```python
from build123d import *

# Parameters (mm, degrees)
F0_R     = 2
F0_R_2   = 2.5
F1_DEPTH = 2
F2_R     = 2
F3_R     = 5
F4_R     = 12
F5_R     = 5
F6_R     = 16


with BuildPart() as f1:
    # F0 (on Top) → F1 (new body)
    with BuildSketch(Plane.XY):
        Polygon((-40.6955056692, 2.5), (-31.6955056692, 2.5), (-31.6955056692, 9.2036510807), (-65, 42.5081454115), (-65, 34.5), (-65, 2.5), align=None)
        with Locations((-40.6955056692, 11.5)):
            Circle(F0_R, mode=Mode.SUBTRACT)
        with Locations((-59, 25.5)):
            Circle(F0_R, mode=Mode.SUBTRACT)
        with BuildLine():
            Line((-44, -28.5), (-26, -28.5))
            Line((-26, -28.5), (-26, -0.5))
            Line((-26, -0.5), (-28.6955056692, -0.5))
            ThreePointArc((-28.6955056692, -0.5), (-30.8168260127, 0.3786796564), (-31.6955056692, 2.5))
            Line((-31.6955056692, 2.5), (-40.6955056692, 2.5))
            Line((-40.6955056692, 2.5), (-65, 2.5))
            ThreePointArc((-65, 2.5), (-65.8786796564, 0.3786796564), (-68, -0.5))
            Line((-68, -0.5), (-68, -3))
            Line((-68, -3), (-66, -3))
            Line((-66, -3), (-66, -10))
            Line((-66, -10), (-68, -10))
            Line((-68, -10), (-68, -19.5))
            Line((-68, -19.5), (-55, -19.5))
            Line((-55, -19.5), (-44, -28.5))
        make_face()
        Polygon((-74, -3), (-68, -3), (-68, -0.5), (-72, -0.5), (-74, -0.5), align=None)
        with BuildLine():
            Line((-81, -19.5), (-68, -19.5))
            Line((-68, -19.5), (-68, -10))
            Line((-68, -10), (-71.5, -10))
            Line((-71.5, -10), (-71.5, -13.5))
            ThreePointArc((-71.5, -13.5), (-74, -16), (-76.5, -13.5))
            Line((-76.5, -13.5), (-76.5, -8.9494897428))
            ThreePointArc((-76.5, -8.9494897428), (-77.2267021942, -5.1441264992), (-74, -3))
            Line((-74, -3), (-74, -0.5))
            Line((-74, -0.5), (-81, -0.5))
            Line((-81, -0.5), (-81, -19.5))
        make_face()
        Polygon((-81, 2.5), (-81, -0.5), (-74, -0.5), (-72, -0.5), (-72, 10.5), (-86, 10.5), (-86, 2.5), align=None)
        with Locations((-79, 6.5)):
            Circle(F0_R, mode=Mode.SUBTRACT)
        with BuildLine():
            ThreePointArc((26, 24.5), (24.8284271247, 27.3284271247), (22, 28.5))
            Line((22, 28.5), (18.5, 28.5))
            Line((18.5, 28.5), (15, 28.5))
            ThreePointArc((15, 28.5), (12.1715728753, 27.3284271247), (11, 24.5))
            Line((11, 24.5), (11, 2.5))
            Line((11, 2.5), (11, 1.4913195046))
            ThreePointArc((11, 1.4913195046), (10, 0.4913195046), (9, 1.4913195046))
            Line((9, 1.4913195046), (9, 2.4990135962))
            Line((9, 2.4990135962), (9, 8.4837929157))
            Line((9, 8.4837929157), (-7.795591982, 28.5))
            Line((-7.795591982, 28.5), (-15.9371936145, 28.5))
            ThreePointArc((-15.9371936145, 28.5), (-16, 28.4990135962), (-16.0628063855, 28.5))
            Line((-16.0628063855, 28.5), (-21, 28.5))
            Line((-21, 28.5), (-21, 10.4990135962))
            Line((-21, 10.4990135962), (-21, 2.4990135962))
            ThreePointArc((-21, 2.4990135962), (-21.8516547202, 0.4050669496), (-23.9230750393, -0.5))
            ThreePointArc((-23.9230750393, -0.5), (-24, -0.5009864038), (-24.0769249607, -0.5))
            Line((-24.0769249607, -0.5), (-26, -0.5))
            Line((-26, -0.5), (-26, -28.5))
            Line((-26, -28.5), (-7, -28.5))
            Line((-7, -28.5), (9, -28.5))
            Line((9, -28.5), (10, -28.5))
            Line((10, -28.5), (11, -28.5))
            Line((11, -28.5), (22, -28.5))
            ThreePointArc((22, -28.5), (24.8284271247, -27.3284271247), (26, -24.5))
            Line((26, -24.5), (26, 24.5))
        make_face()
        with BuildLine():
            ThreePointArc((12.5, -18.5), (11.767766953, -20.267766953), (10, -21))
            ThreePointArc((10, -21), (8.232233047, -16.732233047), (12.5, -18.5))
        make_face(mode=Mode.SUBTRACT)
        with Locations((-7, -9.5)):
            Circle(F0_R_2, mode=Mode.SUBTRACT)
        with BuildLine():
            ThreePointArc((-14, 10.4990135962), (-16, 8.4990135962), (-18, 10.4990135962))
            ThreePointArc((-18, 10.4990135962), (-16, 12.4990135962), (-14, 10.4990135962))
        make_face(mode=Mode.SUBTRACT)
        with BuildLine():
            ThreePointArc((3, 10.4990135962), (1, 8.4990135962), (-1, 10.4990135962))
            ThreePointArc((-1, 10.4990135962), (1, 12.4990135962), (3, 10.4990135962))
        make_face(mode=Mode.SUBTRACT)
        with BuildLine():
            ThreePointArc((21, 14.5), (16.732233047, 12.732233047), (18.5, 17))
            ThreePointArc((18.5, 17), (20.267766953, 16.267766953), (21, 14.5))
        make_face(mode=Mode.SUBTRACT)
        with BuildLine():
            Line((-15.9371936145, 28.5), (-7.795591982, 28.5))
            Line((-7.795591982, 28.5), (-12.1697777844, 33.7129516447))
            ThreePointArc((-12.1697777844, 33.7129516447), (-17.7101007166, 35.1974767002), (-21, 30.4990135962))
            Line((-21, 30.4990135962), (-21, 28.5))
            Line((-21, 28.5), (-16.0628063855, 28.5))
            ThreePointArc((-16.0628063855, 28.5), (-17.3918310294, 31.9352609236), (-14, 30.4990135962))
            ThreePointArc((-14, 30.4990135962), (-14.5637526726, 29.1071825668), (-15.9371936145, 28.5))
        make_face()
    extrude(amount=F1_DEPTH)

    # F2
    f2_edges = [f1.edges().sort_by_distance(p)[0] for p in [
        (-72, 10.5, 1),
        (-86, 10.5, 1),
        (-86, 2.5, 1),
        (-81, 2.5, 1),
        (-72, -0.5, 1),
    ]]
    fillet(f2_edges, radius=F2_R)

    # F3
    f3_edges = [f1.edges().sort_by_distance(p)[0] for p in [
        (-65, 42.508145, 1),
    ]]
    fillet(f3_edges, radius=F3_R)

    # F4
    f4_edges = [f1.edges().sort_by_distance(p)[0] for p in [
        (-31.695506, 9.203651, 1),
        (9, 8.483793, 1),
    ]]
    fillet(f4_edges, radius=F4_R)

    # F5
    f5_edges = [f1.edges().sort_by_distance(p)[0] for p in [
        (-81, -19.5, 1),
    ]]
    fillet(f5_edges, radius=F5_R)

    # F6
    f6_edges = [f1.edges().sort_by_distance(p)[0] for p in [
        (-55, -19.5, 1),
        (-44, -28.5, 1),
    ]]
    fillet(f6_edges, radius=F6_R)


solid = f1.part
```
Input: part model. Units: mm. Frame: model coordinates. A direction names the side the tool comes from. Coordinates: 2 decimals unless noted, no trailing zeros. Write each loop counter-clockwise with the first axis right and the second up, starting at its lowest first coordinate (ties: lowest second). Pieces come first, ordered by that corner, then holes. Notation, with made-up numbers: M 33.25,58 L 58.25,58 A11 cw 58.25,74 Z; hole C 7,80.25 d8. An arc over 180 degrees is marked long. Use one line per item in the form item = value.
Q1. Section C-C (x = -79). Return loops of the section in (y, z), plus the area to 3 significant figures.
Answer below:
outline = M -18.5,0 L 4.5,0 L 4.5,2 L -18.5,2 Z; M 8.5,0 L 10.5,0 L 10.5,2 L 8.5,2 Z
area = 50.0 mm²
Q2. Section A-A (x = -59). Return loops of the section in (y, z).
Answer below:
outline = M -19.59,0 L 23.5,0 L 23.5,2 L -19.59,2 Z; M 27.5,0 L 35.34,0 L 35.34,2 L 27.5,2 Z
Q3. Section D-D (z = 1.3). Count the separate pieces of the cut face and the enclosed holes in it, plus the area to 3 significant figures.
Answer below:
separate_pieces = 1
enclosed_holes = 10
area = 4,650 mm²
Q4. Material intervals for probe 1 along Y at (x, z) = (-16, 1.15); probe 2 along Y at (x, z) = (-79, 0.7); probe 3 along X at (y, z) = (9, 1.2), sorted ascending. Write a range as from..to.
Answer below:
probe_1 = -28.5..8.5, 12.5..28.5, 32.5..35.5
probe_2 = -18.5..4.5, 8.5..10.5
probe_3 = -85.94..-72.06, -65..-32.68, -21..-17.32, -14.68..-0.32, 2.32..7.96, 11..26
Q5. Draft query along Y for faces 4 (the face through (-85.4, 9.93, 1.01)), 5 (the face through (-81, -7, 1)), 6 (the face through (-77.25, -5.2, 0.99)). Return one class per face: released by +Y, released by -Y, zero draft, split by the parting line, or undercut.
Answer below:
face_4 = released by +Y
face_5 = zero draft
face_6 = undercut
Q6. First-contact query: pin 1 (0.8 mm diameter, centred on x = -83.5, z = 1, fed in from -Y); pin 2 (1 mm diameter, centred on x = -68.5, z = 1.5, fed in from +Y); pin 3 (1 mm diameter, centred on x = -80.5, z = 0.5, fed in from +Y). Flat tips, straight axial feed; report the tip coordinate or a pass-through.
Answer below:
pin_1 = 2.5
pin_2 = -0.5
pin_3 = 10.5
Q7. Section B-B (y = 21). Return loops of the section in (x, z).
Answer below:
outline = M -65,0 L -43.49,0 L -43.49,2 L -65,2 Z; M -21,0 L -1.5,0 L -1.5,2 L -21,2 Z; M 11,0 L 26,0 L 26,2 L 11,2 Z
Q8. Set-up query: faces 1 (the face through (-69, -10, 1)), 2 (the face through (11, 13, 1)), 3 (the face through (-79, 10.5, 1)). Return all of +Z, -Z, +X, -X, +Y, -Y with unobstructed straight access to the full face (end or side cutting, diameter ignored); none if empty.
Answer below:
face_1 = +Z, -Z
face_2 = +Z, -Z, +Y
face_3 = +Z, -Z, -X, +Y
